Could you check a few things on this model? Use its own coordinates, in mm. A direction names the side the tool comes from. Give positions to 0.01 mm unless a question says otherwise; leave off trailing zeros. Loops run counter-clockwise (first coordinate to the right, second up) from the corner with the lowest first, then second, coordinate; pieces in that order, holes last. Notation, with made-up numbers: M 67,0.25 L 110,0.25 A9 ccw 110,16.25 Z; hole C 86,-4.75 d11. An arc over 180 degrees is marked long. Answer in a Markdown table with one row per item. Add a question column.
1. If we section it at B-B on z = -60.5: List the corners of the cut face in (x, y) for me, then the cut area to 3 significant figures.
2. I'm going to push flat-ended pins straight in: pin 1 Ø4 at (y, z) = (197.5, -57.5) entering from +X; pin 2 Ø8 at (x, z) = (-44, -82.5) entering from -Y; pin 3 Ø7.5 at (x, y) = (-65.5, 75) entering from -Z. Where does each tip first touch, or does it pass through?
3. I need wall thicknesses on line 1 along Z through (x, y) = (69.5, 0); line 2 along X through (y, z) = (64, 9.5); line 3 along Y through (x, z) = (6, -81). Which ranges of each line are inside material? Lowest first, please. Write a range as from..to.
4. If we section it at D-D on x = 34.5: List the corners of the cut face in (y, z) for me.
5. If we section it at C-C on z = 11: List the corners of the cut face in (x, y) for me.
6. Which directions (+Z, -Z, +X, -X, +Y, -Y) give clear straight access to the entire face, cutting with the end or side of a thin tool? Please do faces 1 (the flat face through (43, 157, -21)), 2 (the flat face through (-68, 52, -30)), 3 (the flat face through (15.5, 200, -36)).
7. If we section it at A-A on y = 135.5: List the corners of the cut face in (x, z) for me, then the cut area to 3 significant figures.
8. Thinking about a two-plate mould opening in Y: for faces 4 (the flat face through (75, 94, -7)), 5 (the flat face through (0, 184.5, -36)), 6 (the flat face through (60.9, 146.8, -72.3)), which applies, released by +Y, released by -Y, zero draft, split by the parting line, or undercut?
```python
from build123d import *

# Parameters (mm, degrees)
BOSS_EXTRUDE1_DEPTH      = 30
BOSS_EXTRUDE1_DEPTH_BACK = 100
SKETCH2_W                = 31
SKETCH2_H                = 31
CUT_EXTRUDE1_DEPTH       = 258.827946507
CUT_EXTRUDE1_DEPTH_BACK  = 258.827946507
CUT_EXTRUDE2_DEPTH       = 258.827946507
CUT_EXTRUDE2_DEPTH_BACK  = 258.827946507
SKETCH4_R                = 15
FILLET1_R                = 30


with BuildPart() as part:
    # Sketch2 → Boss-Extrude1 (new, two sides: drawn at the far end of the back side and taken through both)
    with BuildSketch(Plane.XY.offset(-BOSS_EXTRUDE1_DEPTH_BACK)):
        Polygon((-25.5, 174.5), (25.5, 174.5), (60, 140), (60, -30), (75, -30), (75, 176), (25.5, 225.5), (-25.5, 225.5), (-75, 176), (-75, -30), (-60, -30), (-60, 140), align=None)
        with Locations((0, 200)):
            Rectangle(SKETCH2_W, SKETCH2_H, mode=Mode.SUBTRACT)
    extrude(amount=BOSS_EXTRUDE1_DEPTH + BOSS_EXTRUDE1_DEPTH_BACK)

    # Sketch3 → Cut-Extrude1 (cut, two sides: drawn at the far end of the back side and taken through both)
    with BuildSketch(Plane(origin=(0, 0, 0), x_dir=(0, 0, -1), z_dir=(1, 0, 0)).offset(-CUT_EXTRUDE1_DEPTH_BACK)):
        Polygon((30, -30), (30, 104.5), (100, 174.5), (100, -30), align=None)
    extrude(amount=CUT_EXTRUDE1_DEPTH + CUT_EXTRUDE1_DEPTH_BACK, mode=Mode.SUBTRACT)

    # Sketch4 → Cut-Extrude2 (cut, two sides: drawn at the far end of the back side and taken through both)
    with BuildSketch(Plane(origin=(0, 0, 0), x_dir=(0, 0, -1), z_dir=(1, 0, 0)).offset(-CUT_EXTRUDE2_DEPTH_BACK)):
        Circle(SKETCH4_R)
    extrude(amount=CUT_EXTRUDE2_DEPTH + CUT_EXTRUDE2_DEPTH_BACK, mode=Mode.SUBTRACT)

    # Fillet1
    fillet1_edges = [part.edges().sort_by_distance(p)[0] for p in [
        (67.5, -30, -30),
        (-67.5, -30, -30),
        (-67.5, -30, 30),
        (67.5, -30, 30),
    ]]
    fillet(fillet1_edges, radius=FILLET1_R - 0.0001)  # a hair under: the kernel refuses the full size


solid = part.part
```
Results:
| question | item | result |
|---|---|---|
| 1 | outline | M -75,135 L -60,135 L -60,140 L -25.5,174.5 L 25.5,174.5 L 60,140 L 60,135 L 75,135 L 75,176 L 25.5,225.5 L -25.5,225.5 L -75,176 Z; hole M -15.5,184.5 L 15.5,184.5 L 15.5,215.5 L -15.5,215.5 Z |
| 1 | area | 6,610 mm2 |
| 2 | pin 1 | x = 55.5 |
| 2 | pin 2 | y = 153.72 |
| 2 | pin 3 | z = -30 |
| 3 | line 1 | -30..-15, 15..30 |
| 3 | line 2 | -75..-60, 60..75 |
| 3 | line 3 | 174.5..184.5, 215.5..225.5 |
| 4 | outline | M 165.5,-91 L 174.5,-100 L 216.5,-100 L 216.5,30 L 165.5,30 Z |
| 5 | outline | M -75,-27.91 L -60,-27.91 L -60,-10.2 L -75,-10.2 Z; M -75,10.2 L -60,10.2 L -60,140 L -25.5,174.5 L 25.5,174.5 L 60,140 L 60,10.2 L 75,10.2 L 75,176 L 25.5,225.5 L -25.5,225.5 L -75,176 Z; M 60,-27.91 L 75,-27.91 L 75,-10.2 L 60,-10.2 Z; hole M -15.5,184.5 L 15.5,184.5 L 15.5,215.5 L -15.5,215.5 Z |
| 6 | face 1 | +Z, -Z, -Y |
| 6 | face 2 | -Z, +X, -X, -Y |
| 6 | face 3 | +Z, -Z |
| 7 | outline | M -75,-61 L -60,-61 L -60,30 L -75,30 Z; M 60,-61 L 75,-61 L 75,30 L 60,30 Z |
| 7 | area | 2,730 mm2 |
| 8 | face 4 | zero draft |
| 8 | face 5 | undercut |
| 8 | face 6 | released by -Y |
